Solid Edge part; units mm, degrees
sketch "Sketch1" plane through (0, 0, 0) normal (0, 0, 1) x (1, 0, 0)
  line L0 (68.9286, 131.9643) -> (188.9286, 131.9643)
  line L1 (188.9286, 131.9643) -> (188.9286, 11.9643)
  line L2 (188.9286, 11.9643) -> (68.9286, 11.9643)
  line L3 (68.9286, 11.9643) -> (68.9286, 131.9643)
  dimension "D1" = 68.9286
  dimension "D2" = 188.9286
  dimension "D3" = 68.9286
extrude "Protrusion1" add sketch "Sketch1" along normal blind 2
sketch "Sketch2" plane through (128.9286, 71.9643, 2) normal (0, 0, 1) x (1, 0, 0)
  circle A0 centre (0, 0) radius 2
extrude "Cutout1" cut sketch "Sketch2" against normal through all
sketch "Sketch3" plane through (128.9286, 71.9643, 2) normal (0, 0, 1) x (1, 0, 0)
  circle A0 centre (0, 0) radius 3.25
extrude "ExtrudedCutout_3" cut sketch "Sketch3" against normal blind 1
Geometry: final body of the model. Coordinates: model frame, mm. A direction names the side the tool comes from. Round coordinates to 2 decimals unless told otherwise and drop trailing zeros. Write item = value, one per line. Start each with the question number.
Q1. Access query for faces 3 (the flat face through (127, 71, 1)), 4 (the flat face through (130, 86, 2)). Directions: +Z, -Z, +X, -X, +Y, -Y. A direction counts if a zero-diameter tool reaches every point of the face in a straight line with its end or side. Return the directions, or none.
Q2. Pull-direction query (X, two-part tool) for faces 1 (the cylindrical face through (131.93, 70.72, 1.51)), 2 (the flat face through (130, 86, 0)); classes: +X half, -X half, draft (parallel to the pull), parting line (faces both ways), or undercut.
Q3. Pin query (flat end, axial travel): pin 1 (5 mm diameter, centred on x = 128.93, y = 71.96, fed in from +Z). Return the tip coordinate at first contact, or that it passes through.
Outcome:
q1.face_3 = +Z
q1.face_4 = +Z, +X, -X, +Y, -Y
q2.face_1 = undercut
q2.face_2 = draft
q3.pin_1 = 1
